from build123d import *

# Parameters (mm, degrees)
BOSS_EXTRUDE1_DEPTH          = 3
SKETCH2_W                    = 10
SKETCH2_H                    = 416.9
BOSS_EXTRUDE2_DEPTH          = 0.1
CUT_EXTRUDE1_DEPTH           = 10
M3_CLEARANCE_HOLE1_OUTLINE_R = 1.6
M3_CLEARANCE_HOLE1_DEPTH     = 3
M3_CLEARANCE_HOLE2_OUTLINE_R = 1.7
M3_CLEARANCE_HOLE2_DEPTH     = 3
SKETCH6_W                    = 5
SKETCH6_H                    = 296.9
CUT_EXTRUDE2_DEPTH           = 10
MOVE_FACE1_BY                = 0.8
MOVE_FACE1_2_BY              = 0.8
MOVE_FACE1_3_BY              = 0.8
MOVE_FACE1_4_BY              = 0.8
MOVE_FACE1_5_BY              = 0.8
MOVE_FACE1_6_BY              = 0.8
MOVE_FACE1_7_BY              = 0.8
MOVE_FACE1_8_BY              = 0.8


# Read off the part's stored shape, not the designer's step: M3 Clearance Hole1, M3 Clearance Hole2
with BuildPart() as part:
    # Sketch1 → Boss-Extrude1 (new body)
    with BuildSketch(Plane.XY):
        Polygon((0, 0), (136, 0), (136, 120), (300, 120), (300, 416.9), (0, 416.9), align=None)
    extrude(amount=BOSS_EXTRUDE1_DEPTH)


with BuildPart() as body_2:
    # Sketch2 → Boss-Extrude2 (new body)
    with BuildSketch(Plane.XY):
        with Locations((1, 208.45)):
            Rectangle(SKETCH2_W, SKETCH2_H)
    extrude(amount=-BOSS_EXTRUDE2_DEPTH)


with BuildPart() as cut_extrude1_tool:
    # Sketch3 → Cut-Extrude1 (new body)
    with BuildSketch(Plane.XY.offset(3)):
        Polygon((0, 416.9), (-4, 416.9), (-4, 396.9), (0, 396.9), (12, 396.9), (12, 416.9), align=None)
        Polygon((0, 0), (12, 0), (12, 20), (0, 20), (-4, 20), (-4, 0), align=None)
    extrude(amount=-CUT_EXTRUDE1_DEPTH)


with BuildPart() as part_1:
    add(part.part)

    # Cut-Extrude1: cut by cut_extrude1_tool
    add(cut_extrude1_tool.part, mode=Mode.SUBTRACT)

    # M3 Clearance Hole1 outline → M3 Clearance Hole1 (cut)
    with BuildSketch(Plane.XY):
        with Locations((31, 30)):
            Circle(M3_CLEARANCE_HOLE1_OUTLINE_R)
        with Locations((19, 30)):
            Circle(M3_CLEARANCE_HOLE1_OUTLINE_R)
        with Locations((31, 386.9)):
            Circle(M3_CLEARANCE_HOLE1_OUTLINE_R)
        with Locations((19, 386.9)):
            Circle(M3_CLEARANCE_HOLE1_OUTLINE_R)
    extrude(amount=M3_CLEARANCE_HOLE1_DEPTH, mode=Mode.SUBTRACT)

    # M3 Clearance Hole2 outline → M3 Clearance Hole2 (cut)
    with BuildSketch(Plane.XY):
        with Locations((271, 178.45)):
            Circle(M3_CLEARANCE_HOLE2_OUTLINE_R)
        with Locations((271, 238.45)):
            Circle(M3_CLEARANCE_HOLE2_OUTLINE_R)
    extrude(amount=M3_CLEARANCE_HOLE2_DEPTH, mode=Mode.SUBTRACT)

    # Sketch6 → Cut-Extrude2 (cut)
    with BuildSketch(Plane.XY.offset(3)):
        with Locations((297.5, 268.45)):
            Rectangle(SKETCH6_W, SKETCH6_H)
    extrude(amount=-CUT_EXTRUDE2_DEPTH, mode=Mode.SUBTRACT)

    # Move Face1: a face moved inward by 0.8
    extrude(part_1.faces().sort_by_distance((215.5, 120, 1.5))[0], amount=MOVE_FACE1_BY, dir=(0, 1, 0), mode=Mode.SUBTRACT)

    # Move Face1 2: a face moved inward by 0.8
    extrude(part_1.faces().sort_by_distance((136, 60, 1.5))[0], amount=MOVE_FACE1_2_BY, dir=(-1, 0, 0), mode=Mode.SUBTRACT)

    # Move Face1 3: a face moved inward by 0.8
    extrude(part_1.faces().sort_by_distance((74, 0, 1.5))[0], amount=MOVE_FACE1_3_BY, dir=(0, 1, 0), mode=Mode.SUBTRACT)

    # Move Face1 4: a face moved inward by 0.8
    extrude(part_1.faces().sort_by_distance((12, 10, 1.5))[0], amount=MOVE_FACE1_4_BY, dir=(1, 0, 0), mode=Mode.SUBTRACT)

    # Move Face1 5: a face moved inward by 0.8
    extrude(part_1.faces().sort_by_distance((6, 20, 1.5))[0], amount=MOVE_FACE1_5_BY, dir=(0, 1, 0), mode=Mode.SUBTRACT)

    # Move Face1 6: a face moved inward by 0.8
    extrude(part_1.faces().sort_by_distance((153.5, 416.9, 1.5))[0], amount=MOVE_FACE1_6_BY, dir=(0, -1, 0), mode=Mode.SUBTRACT)

    # Move Face1 7: a face moved inward by 0.8
    extrude(part_1.faces().sort_by_distance((12, 406.9, 1.5))[0], amount=MOVE_FACE1_7_BY, dir=(1, 0, 0), mode=Mode.SUBTRACT)

    # Move Face1 8: a face moved inward by 0.8
    extrude(part_1.faces().sort_by_distance((6, 396.9, 1.5))[0], amount=MOVE_FACE1_8_BY, dir=(0, -1, 0), mode=Mode.SUBTRACT)


with BuildPart() as body_2_1:
    add(body_2.part)

    # Cut-Extrude1: cut by cut_extrude1_tool
    add(cut_extrude1_tool.part, mode=Mode.SUBTRACT)


solid = part_1.part
Here's how the part is built. I have some questions about the finished solid (model axes, mm). Give positions to 0.01 mm unless a question says otherwise; leave off trailing zeros. Loops run counter-clockwise (first coordinate to the right, second up) from the corner with the lowest first, then second, coordinate; pieces in that order, holes last. Notation, with made-up numbers: (-32, -16) -> (1, -16) arc R28 ccw to (1, 8) -> close; hole circle Ø2 at (66.25, 8). An arc over 180 degrees is marked (long way). Answer as a JSON object with one key per item and string values. Group by question number.
Item 1: Imagine slicing it at A-A on z = 1.7. Write out the boundary of the cut face in (x, y), then the cut area to 3 significant figures.
Item 2: I need wall thicknesses on L1, parallel to Y at x = 19, z = 1.95; L2, parallel to X at y = 386.9, z = 0.6; L3, parallel to X at y = 178.45, z = 1.35. Which ranges of each line are inside material? Lowest first, please.
Item 3: Imagine slicing it at C-C on x = 250.5. Write out the boundary of the cut face in (y, z).
Item 4: Will these pins go through, and if not, where does the flat tip stop? pin 1 (1.5 mm diameter, centred on x = 4.5, z = 2, fed in from -Y); pin 2 (5 mm diameter, centred on x = 31, y = 386.9, fed in from +Z); pin 3 (1.5 mm diameter, centred on x = 6, z = 1.5, fed in from +Y); pin 4 (1.5 mm diameter, centred on y = 408, z = 1.5, fed in from -X).
Item 5: Imagine slicing it at B-B on y = 112. Write out the boundary of the cut face in (x, z).
Answer list:
{
 "1": {"outline": "(0, 20.8) -> (12.8, 20.8) -> (12.8, 0.8) -> (135.2, 0.8) -> (135.2, 120.8) -> (295, 120.8) -> (295, 416.1) -> (12.8, 416.1) -> (12.8, 396.1) -> (0, 396.1) -> close; hole circle Ø3.2 at (19, 30); hole circle Ø3.2 at (19, 386.9); hole circle Ø3.2 at (31, 30); hole circle Ø3.2 at (31, 386.9); hole circle Ø3.4 at (271, 178.45); hole circle Ø3.4 at (271, 238.45)", "area": "103,000 mm2"},
 "2": {"L1": "y = 0.8 to 28.4, 31.6 to 385.3, 388.5 to 416.1", "L2": "x = 0 to 17.4, 20.6 to 29.4, 32.6 to 295", "L3": "x = 0 to 269.3, 272.7 to 295"},
 "3": {"outline": "(120.8, 0) -> (416.1, 0) -> (416.1, 3) -> (120.8, 3) -> close"},
 "4": {"pin 1": "stops at y = 20.8", "pin 2": "stops at z = 3", "pin 3": "stops at y = 396.1", "pin 4": "stops at x = 12.8"},
 "5": {"outline": "(0, 0) -> (135.2, 0) -> (135.2, 3) -> (0, 3) -> close"}
}
